Verification items for the finished model (mm, model axes). A direction names the side the tool comes from. Round coordinates to 2 decimals unless told otherwise and drop trailing zeros. Loops run counter-clockwise (first coordinate to the right, second up) from the corner with the lowest first, then second, coordinate; pieces in that order, holes last. Notation, with made-up numbers: (-21, 59) -> (11, 59) arc R7 ccw to (11, 63) -> close; hole circle Ø8 at (62, 20.25). An arc over 180 degrees is marked (long way). Write item = value, one per line.
```python
from build123d import *

# Parameters (mm, degrees)
SKETCH_R          = 1
EXTRUDE_DEPTH     = 13
BOX002_W          = 1.6
BOX002_H          = 15
BOX002_DEPTH      = 12
CYLINDER007_R     = 2
CYLINDER007_DEPTH = 22
CYLINDER006_R     = 3.2
CYLINDER006_DEPTH = 15
CYLINDER005_R     = 10.63
CYLINDER005_DEPTH = 41


with BuildPart() as servoholes001:
    # Sketch → Extrude (new body)
    with BuildSketch(Plane.XZ):
        with Locations((11.094024, 19.711318)):
            Circle(SKETCH_R)
        with Locations((25.094024, 19.711318)):
            Circle(SKETCH_R)
        with Locations((18.156256, 26.77355)):
            Circle(SKETCH_R)
        with Locations((18.156256, 12.77355)):
            Circle(SKETCH_R)
    extrude(amount=EXTRUDE_DEPTH)


with BuildPart() as servoholes001_1:
    # Extrude placement: moved
    add(servoholes001.part.moved(Location((0, 32, 0))))


with BuildPart() as slit002:
    # Box002 → Box002 (new body)
    with BuildSketch(Plane(origin=(17.3, 45, 13.8), x_dir=(1, 0, 0), z_dir=(0, 0, 1))):
        with Locations((0.8, 7.5)):
            Rectangle(BOX002_W, BOX002_H)
    extrude(amount=BOX002_DEPTH)


with BuildPart() as bolthole001:
    # Cylinder007 → Cylinder007 (new body)
    with BuildSketch(Plane(origin=(18, 55, 9), x_dir=(1, 0, 0), z_dir=(0, 0, 1))):
        Circle(CYLINDER007_R)
    extrude(amount=CYLINDER007_DEPTH)


with BuildPart() as inner001:
    # Cylinder006 → Cylinder006 (new body)
    with BuildSketch(Plane(origin=(18, 60, 20), x_dir=(1, 0, 0), z_dir=(0, -1, 0))):
        Circle(CYLINDER006_R)
    extrude(amount=CYLINDER006_DEPTH)

    # Fusion003: union slit002, boltHole001
    add(slit002.part)
    add(bolthole001.part)


with BuildPart() as connect001:
    # Cylinder005 → Cylinder005 (new body)
    with BuildSketch(Plane(origin=(18, 60, 20), x_dir=(1, 0, 0), z_dir=(0, -1, 0))):
        Circle(CYLINDER005_R)
    extrude(amount=CYLINDER005_DEPTH)

    # Cut002: cut inner001
    add(inner001.part, mode=Mode.SUBTRACT)

    # Cut003: cut servoHoles001
    add(servoholes001_1.part, mode=Mode.SUBTRACT)


solid = connect001.part
```
(1) Sectioned sample at A-A, the plane y = 55. Record the cut outline in (x, z).
Filled sheet:
outline = (16, 9.56) -> (16, 17.5) arc R3.2 cw to (16, 22.5) -> (16, 30.44) arc R10.63 ccw to start; (20, 9.56) arc R10.63 ccw to (20, 30.44) -> (20, 22.5) arc R3.2 cw to (20, 17.5) -> close
(2) Go/stop test with flat-tipped pins: pin 1 Ø1.5 at (y, z) = (35, 15) entering from -X; pin 2 Ø4 at (x, y) = (22.5, 53.5) entering from -Z; pin 3 Ø3 at (y, z) = (58.5, 24.5) entering from -X. Record where each tip stops, or that it passes through.
Filled sheet:
pin_1 = 8.26
pin_2 = 9.67
pin_3 = 7.8
(3) Sectioned sample at D-D, the plane z = 28.5. Record the cut outline in (x, y), and give its area (3 significant figures).
Filled sheet:
outline = (11.62, 19) -> (24.38, 19) -> (24.38, 60) -> (11.62, 60) -> close; hole circle Ø4 at (18, 55)
area = 511 mm2
(4) Material ranges on probe 1 along Z at (x, y) = (18.75, 27); probe 2 along X at (y, z) = (55, 26.75); probe 3 along Z at (x, y) = (17.75, 23.5), recorded low to high. Write a range as from..to.
Filled sheet:
probe_1 = 9.4..11.97, 13.58..25.97, 27.58..30.6
probe_2 = 9.79..16, 20..26.21
probe_3 = 9.37..11.86, 13.69..25.86, 27.69..30.63
(5) Sectioned sample at C-C, the plane y = 46.5. Record the cut outline in (x, z), and give its area (3 significant figures).
Filled sheet:
outline = circle Ø21.26 at (18, 20); hole (17.3, 13.8) -> (18.9, 13.8) -> (18.9, 16.93) arc R3.2 ccw to (18.9, 23.07) -> (18.9, 25.8) -> (17.3, 25.8) -> (17.3, 23.12) arc R3.2 ccw to (17.3, 16.88) -> close
area = 314 mm2
(6) Set-up check for faces 4 (the face through (20, 60, 23)), 5 (the face through (17.939, 25.591, 11.797)), 6 (the face through (18.9, 58, 24)): record each of +Z, -Z, +X, -X, +Y, -Y from which the full face is reachable in a straight line by a thin tool's end or side.
Filled sheet:
face_4 = +Z, -Z, +X, -X, +Y
face_5 = -Y
face_6 = +Y
(7) Sectioned sample at B-B, the plane x = 18. Record the cut outline in (y, z).
Filled sheet:
outline = (19, 9.37) -> (53, 9.37) -> (53, 13.8) -> (45, 13.8) -> (45, 25.8) -> (53, 25.8) -> (53, 30.63) -> (19, 30.63) -> (19, 27.76) -> (32, 27.76) -> (32, 25.79) -> (19, 25.79) -> (19, 13.76) -> (32, 13.76) -> (32, 11.79) -> (19, 11.79) -> close; (57, 9.37) -> (60, 9.37) -> (60, 13.8) -> (57, 13.8) -> close; (57, 25.8) -> (60, 25.8) -> (60, 30.63) -> (57, 30.63) -> close
(8) Draft check along Y on faces 1 (the face through (18, 45, 20)), 2 (the face through (18, 58, 13.8)), 3 (the face through (19.847, 54.234, 26.51)). Enter one of: released by +Y, released by -Y, zero draft, split by the parting line, or undercut.
Filled sheet:
face_1 = released by +Y
face_2 = zero draft
face_3 = undercut
